The model under review builds one solid part; all positions refer to its coordinate system, in mm. A direction names the side the tool comes from. Coordinates: 2 decimals unless noted, no trailing zeros. Loops run counter-clockwise (first coordinate to the right, second up) from the corner with the lowest first, then second, coordinate; pieces in that order, holes last. Notation, with made-up numbers: (22.25, -23) - (75.25, -23) arc R11 cw to (75.25, -7) - close; hole circle Ø6 at (29.5, 4). An arc over 180 degrees is marked (long way). One line per item, written item: value. Start each with the question number.
1. Mouldability with a two-part tool opening along Y and no side actions: class faces 1 (the face through (250, -240, 227)), 2 (the face through (-3, -230, 690)) as +Y half, -Y half, draft (parallel to the pull), parting line (faces both ways), or undercut.
2. We need section B-B, the plane x = -86. Give the boundary of the cut face in (y, z), then the cut area to 3 significant figures.
3. We need section C-C, the plane z = 161. Give the boundary of the cut face in (x, y), then the cut area to 3 significant figures.
4. Insertion check: P1, Ø6, axis at x = -74.5, y = -235.5, coming from the -Z side. The pin has a flat end and moves straight along its axis. Give the tip position at first contact, or say it passes through.
5. We need section A-A, the plane y = -99. Give the boundary of the cut face in (x, z), then the cut area to 3 significant figures.
6. To check wall thickness, follow line 1 (X direction, y = -198, z = -4.5); line 2 (Y direction, x = -163.5, z = -8). State the ranges of each line that lie inside material, in increasing order.
7. For faces 3 (the face through (-3, 230, 690)), 4 (the face through (-260, 3, 0)), 5 (the face through (3, 240, 460)), 6 (the face through (-21, -240, 700)), 7 (the face through (-260, 4, -40)), list the 3-axis set-ups (+Z, -Z, +X, -X, +Y, -Y) from which the entire face can be reached by the end or side of a thin tool; tool diameter is ignored.
from build123d import *

# Parameters (mm, degrees)
F0_W          = 540
F0_H          = 500
F1_DEPTH      = 700
F1_DEPTH_BACK = 40
F2_W          = 500
F2_H          = 20
F3_DEPTH      = 500.001
F4_W          = 500
F4_H          = 200
F5_DEPTH      = 500.001
F6_W          = 460
F6_H          = 200
F7_DEPTH      = 540.001
F8_W          = 500
F8_H          = 460
F9_DEPTH      = 740.001
F10_W         = 500
F10_H         = 460
F11_DEPTH     = 500.001
F12_W         = 460
F12_H         = 460
F13_DEPTH     = 540.001


with BuildPart() as f1:
    # F0 (on Top) → F1 (new body, two sides)
    with BuildSketch(Plane.XY) as f1_sk:
        Rectangle(F0_W, F0_H)
    extrude(amount=F1_DEPTH)
    extrude(f1_sk.sketch, amount=-F1_DEPTH_BACK)

    # F2 (on face) → F3 (cut, through all)
    with BuildSketch(Plane.XZ.offset(250)):
        with Locations((0, -30)):
            Rectangle(F2_W, F2_H)
    extrude(amount=-F3_DEPTH, mode=Mode.SUBTRACT)

    # F4 (on face) → F5 (cut, through all)
    with BuildSketch(Plane.XZ.offset(250)):
        with Locations((0, 580)):
            Rectangle(F4_W, F4_H)
    extrude(amount=-F5_DEPTH, mode=Mode.SUBTRACT)

    # F6 (on face) → F7 (cut, through all)
    with BuildSketch(Plane(origin=(-270, 0, 0), x_dir=(0, -1, 0), z_dir=(-1, 0, 0))):
        with Locations((0, 580)):
            Rectangle(F6_W, F6_H)
    extrude(amount=-F7_DEPTH, mode=Mode.SUBTRACT)

    # F8 (on face) → F9 (cut, through all)
    with BuildSketch(Plane.XY.offset(700)):
        Rectangle(F8_W, F8_H)
    extrude(amount=-F9_DEPTH, mode=Mode.SUBTRACT)

    # F10 (on face) → F11 (cut, through all)
    with BuildSketch(Plane(origin=(0, 250, 0), x_dir=(-1, 0, 0), z_dir=(0, 1, 0))):
        with Locations((0, 230)):
            Rectangle(F10_W, F10_H)
    extrude(amount=-F11_DEPTH, mode=Mode.SUBTRACT)

    # F12 (on face) → F13 (cut, through all)
    with BuildSketch(Plane(origin=(-270, 0, 0), x_dir=(0, -1, 0), z_dir=(-1, 0, 0))):
        with Locations((0, 230)):
            Rectangle(F12_W, F12_H)
    extrude(amount=-F13_DEPTH, mode=Mode.SUBTRACT)


solid = f1.part
Findings below:
1. face 1: draft
1. face 2: undercut
2. outline: (-250, -20) - (-230, -20) - (-230, 0) - (-250, 0) - close; (-250, 460) - (-230, 460) - (-230, 480) - (-250, 480) - close; (-250, 680) - (-230, 680) - (-230, 700) - (-250, 700) - close; (230, -20) - (250, -20) - (250, 0) - (230, 0) - close; (230, 460) - (250, 460) - (250, 480) - (230, 480) - close; (230, 680) - (250, 680) - (250, 700) - (230, 700) - close
2. area: 2,400 mm2
3. outline: (-270, -250) - (-250, -250) - (-250, -230) - (-270, -230) - close; (-270, 230) - (-250, 230) - (-250, 250) - (-270, 250) - close; (250, -250) - (270, -250) - (270, -230) - (250, -230) - close; (250, 230) - (270, 230) - (270, 250) - (250, 250) - close
3. area: 1,600 mm2
4. P1: z = -20
5. outline: (-270, -40) - (-250, -40) - (-250, 0) - (-270, 0) - close; (-270, 460) - (-250, 460) - (-250, 480) - (-270, 480) - close; (-270, 680) - (-250, 680) - (-250, 700) - (-270, 700) - close; (250, -40) - (270, -40) - (270, 0) - (250, 0) - close; (250, 460) - (270, 460) - (270, 480) - (250, 480) - close; (250, 680) - (270, 680) - (270, 700) - (250, 700) - close
5. area: 3,200 mm2
6. line 1: -270 to -250, 250 to 270
6. line 2: -250 to -230, 230 to 250
7. face 3: +Z, -Z
7. face 4: +X, -X
7. face 5: +Y, -Y
7. face 6: +Z, +X, -X, +Y, -Y
7. face 7: -Z, +X, -X, +Y, -Y
